Can you work these out from the model? Positions are in its coordinate system, mm. Coordinates: 2 decimals unless noted, no trailing zeros. Loops run counter-clockwise (first coordinate to the right, second up) from the corner with the lowest first, then second, coordinate; pieces in that order, holes last.
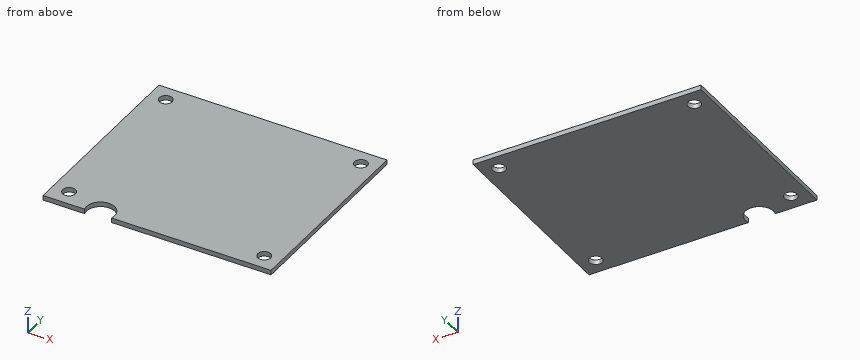
```python
from build123d import *

# Parameters (mm, degrees)
F0_W     = 97
F0_H     = 84
F1_DEPTH = 2
F2_R     = 2.75
F3_DEPTH = 2
F5_DEPTH = 2


with BuildPart() as f1:
    # F0 (on Top) → F1 (new body)
    with BuildSketch(Plane.XY):
        Rectangle(F0_W, F0_H)
    extrude(amount=F1_DEPTH)

    # F2 (on face) → F3 (cut, through all)
    with BuildSketch(Plane.XY.offset(2)):
        with Locations((-41.504115, 35.0012)):
            Circle(F2_R)
        with Locations((41.504115, 35.0012)):
            Circle(F2_R)
        with Locations((41.504115, -35.0012)):
            Circle(F2_R)
        with Locations((-41.504115, -35.0012)):
            Circle(F2_R)
    extrude(amount=-F3_DEPTH, mode=Mode.SUBTRACT)

    # F4 (on face) → F5 (cut, through all)
    with BuildSketch(Plane.XY.offset(2)):
        with BuildLine():
            Line((-30.815778, -42), (-19.381491, -42))
            ThreePointArc((-19.381491, -42), (-25.098634, -34.179487), (-30.815778, -42))
        make_face()
    extrude(amount=-F5_DEPTH, mode=Mode.SUBTRACT)


solid = f1.part
```
Item 1: I'm going to push flat-ended pins straight in: P1, Ø9, axis at x = 41.5, y = 35, coming from the -Z side; P2, Ø5, axis at x = -41.5, y = 35, coming from the -Z side. Where does each tip first touch, or does it pass through?
Results are:
P1: stops at z = 0
P2: passes through
Item 2: I need wall thicknesses on line 1 along X through (y, z) = (35, 1); line 2 along Y through (x, z) = (-41.5, 1.55); line 3 along Y through (x, z) = (42.5, 0.65). Which ranges of each line are inside material? Lowest first, please.
Results are:
line 1: x = -48.5 to -44.25, -38.75 to 38.75, 44.25 to 48.5
line 2: y = -42 to -37.75, -32.25 to 32.25, 37.75 to 42
line 3: y = -42 to -37.56, -32.44 to 32.44, 37.56 to 42
Item 3: Suppose I cut it at B-B, the plane z = 1.6. Please give me the cut outline in (x, y), plus the area to 3 significant figures.
Results are:
outline: (-48.5, -42) - (-30.82, -42) arc R6 cw (long way) to (-19.38, -42) - (48.5, -42) - (48.5, 42) - (-48.5, 42) - close; hole circle Ø5.5 at (-41.5, -35); hole circle Ø5.5 at (-41.5, 35); hole circle Ø5.5 at (41.5, -35); hole circle Ø5.5 at (41.5, 35)
area: 7,970 mm2
Item 4: Suppose I cut it at A-A, the plane x = -42. Please give me the cut outline in (y, z), plus the area to 3 significant figures.
Results are:
outline: (-42, 0) - (-37.71, 0) - (-37.71, 2) - (-42, 2) - close; (-32.3, 0) - (32.3, 0) - (32.3, 2) - (-32.3, 2) - close; (37.71, 0) - (42, 0) - (42, 2) - (37.71, 2) - close
area: 146 mm2
